For this review, take the finished solid that the model builds, in its own axes (mm). A direction names the side the tool comes from. Coordinates: 2 decimals unless noted, no trailing zeros. Write each loop counter-clockwise with the first axis right and the second up, starting at its lowest first coordinate (ties: lowest second). Pieces come first, ordered by that corner, then holes. Notation, with made-up numbers: (-14, 16) -> (-6, 16) arc R6 cw to (-6, 25) -> close; hole circle Ø1 at (-24.5, 44.25). An arc over 180 degrees is marked (long way). Put each result on its own line as item: value. Start each with the question number.
Item 1: Consider section B-B on x = 0. Give the boundary of the cut face in (y, z), and give its area (3 significant figures).
Item 2: To check wall thickness, follow L1, parallel to X at y = 26.5, z = -99.25; L2, parallel to X at y = 38.5, z = -103; L3, parallel to X at y = 75, z = -90.75. State the ranges of each line that lie inside material, in increasing order.
Item 3: For faces 1 (the cylindrical face through (0.45, 90.24, -98.56)), 2 (the flat face through (38.1, 25, -98)), 3 (the conical face through (-1.04, 77.767, -98.292)), 4 (the flat face through (20.396, 51, -99)), 5 (the flat face through (-20.396, 51, -99)), list the 3-axis set-ups (+Z, -Z, +X, -X, +Y, -Y) from which the entire face can be reached by the end or side of a thin tool; tool diameter is ignored.
Item 4: Insertion check: P1, Ø8, axis at x = -29.25, z = -98.42, coming from the +Y side; P2, Ø5.5, axis at y = 55, z = -97, coming from the +X side; P3, Ø4, axis at x = -2.5, z = -100, coming from the +Y side. Each pin has a flat end and moves straight along its axis. Give the tip position at first contact, or say it passes through.
Item 5: Consider section D-D on z = -99.75. Give the number of separate pieces and of enclosed holes in the cut face, and give its area (3 significant figures).
Item 6: Consider section A-A on z = -106.5. Give the boundary of the cut face in (x, y), and give its area (3 significant figures).
Item 7: The part is to be moulded in two halves that separate along Z. For faces 6 (the flat face through (25, 31.75, -94)), 7 (the flat face through (-1, 46, -107.95)), 8 (the cylindrical face through (-31.592, 24.058, -99.163)), 9 (the cylindrical face through (28.114, 24.058, -96.245)), say which applies: +Z half, -Z half, draft (parallel to the pull), parting line (faces both ways), or undercut.
Item 8: Consider section C-C on y = 25.5. Give the boundary of the cut face in (x, z) (3 decimals), and give its area (3 significant figures).
```python
from build123d import *

# Parameters (mm, degrees)
SKETCH1_W                                         = 76.2
SKETCH1_H                                         = 19.05
BOSS_EXTRUDE1_DEPTH                               = 104.14
CUT_EXTRUDE1_DEPTH                                = 131.346801265
CSK_FOR_8_FLAT_HEAD_MACHINE_SCREW_100_D           = 4.9149
CSK_FOR_8_FLAT_HEAD_MACHINE_SCREW_100_CSINK_D     = 10.9728
CSK_FOR_8_FLAT_HEAD_MACHINE_SCREW_100_CSINK_ANGLE = 100


# Read off the part's stored shape, not the designer's step: SurfaceCut1
with BuildPart() as part:
    # Sketch1 → Boss-Extrude1 (new body)
    with BuildSketch(Plane(origin=(0, 19.05, 0), x_dir=(1, 0, 0), z_dir=(0, 1, 0))):
        with Locations((0, 98.425)):
            Rectangle(SKETCH1_W, SKETCH1_H)
    extrude(amount=BOSS_EXTRUDE1_DEPTH)

    # SurfaceCut1 outline → SurfaceCut1 (revolve, cut)
    with BuildSketch(Plane.XZ.offset(-69.85)):
        Polygon((8.266242493, -88.9), (0, -88.9), (0, -107.95), (7.696303968, -107.95), align=None)
    revolve(axis=Axis((0, 69.85, 0), (0, 0, 1)), mode=Mode.SUBTRACT)

    # Sketch3 → Cut-Extrude1 (cut, through all)
    with BuildSketch(Plane(origin=(0, 0, -107.95), x_dir=(-1, 0, 0), z_dir=(0, 0, -1))):
        with BuildLine():
            Line((25.4, 31.75), (37.1816, 31.75))
            Line((37.1816, 31.75), (38.1, 31.75))
            Line((38.1, 31.75), (38.1, 123.19))
            Line((38.1, 123.19), (-38.1, 123.19))
            Line((-38.1, 123.19), (-38.1, 31.75))
            Line((-38.1, 31.75), (-37.1816, 31.75))
            Line((-37.1816, 31.75), (-25.4, 31.75))
            Line((-25.4, 31.75), (-20.396303968, 31.75))
            Line((-20.396303968, 31.75), (-20.396303968, 69.85))
            ThreePointArc((-20.396303968, 69.85), (0, 90.246303968), (20.396303968, 69.85))
            Line((20.396303968, 69.85), (20.396303968, 31.75))
            Line((20.396303968, 31.75), (25.4, 31.75))
        make_face()
    extrude(amount=-CUT_EXTRUDE1_DEPTH, mode=Mode.SUBTRACT)

    # CSK for #8 Flat Head Machine Screw (100)1 (through all)
    with Locations(Plane(origin=(0, 31.75, 0), x_dir=(1, 0, 0), z_dir=(0, 1, 0))):
        with Locations((-29.248151984, 98.425), (29.248151984, 98.425)):
            CounterSinkHole(CSK_FOR_8_FLAT_HEAD_MACHINE_SCREW_100_D / 2, CSK_FOR_8_FLAT_HEAD_MACHINE_SCREW_100_CSINK_D / 2, counter_sink_angle=CSK_FOR_8_FLAT_HEAD_MACHINE_SCREW_100_CSINK_ANGLE)


solid = part.part
```
Return value:
1. outline: (19.05, -107.95) -> (62.15, -107.95) -> (61.58, -88.9) -> (19.05, -88.9) -> close; (77.55, -107.95) -> (90.25, -107.95) -> (90.25, -88.9) -> (78.12, -88.9) -> close
1. area: 1,050 mm^2
2. L1: -38.1 to -31.56, -26.93 to 26.93, 31.56 to 38.1
2. L2: -20.4 to 20.4
2. L3: -19.74 to -6.4, 6.4 to 19.74
3. face 1: +Z, -Z, +Y
3. face 2: +Z, -Z, +X, +Y, -Y
3. face 3: +Z
3. face 4: +Z, -Z, +X, +Y
3. face 5: +Z, -Z, -X, +Y
4. P1: y = 30.51
4. P2: x = 20.4
4. P3: y = 90.24
5. separate pieces: 3
5. enclosed holes: 1
5. area: 2,860 mm^2
6. outline: (-38.1, 19.05) -> (38.1, 19.05) -> (38.1, 31.75) -> (20.4, 31.75) -> (20.4, 69.85) arc R20.4 ccw to (-20.4, 69.85) -> (-20.4, 31.75) -> (-38.1, 31.75) -> close; hole circle Ø15.48 at (0, 69.85)
6. area: 2,990 mm^2
7. face 6: draft
7. face 7: -Z half
7. face 8: undercut
7. face 9: undercut
8. outline: (-38.1, -107.95) -> (38.1, -107.95) -> (38.1, -88.9) -> (-38.1, -88.9) -> close; hole circle Ø4.915 at (-29.248, -98.425); hole circle Ø4.915 at (29.248, -98.425)
8. area: 1,410 mm^2
